Design review of the part shown in the three views and the two pictorial views. Dimensions are in mm from the part's minimum x, y and z. Coordinates: 2 decimals unless noted, no trailing zeros. Loops run counter-clockwise (first coordinate to the right, second up) from the corner with the lowest first, then second, coordinate; pieces in that order, holes last. Notation, with made-up numbers: M 65.25,41.5 L 97.25,41.5 A15 cw 97.25,55.5 Z; hole C 36.5,8.25 d8. An arc over 180 degrees is marked long. Answer as a JSON object with one key per item and string values. Group by question number.
Item 1: Insertion check: pin 1 (3 mm diameter, centred on x = 80.5, y = 5, fed in from -Z); pin 2 (3 mm diameter, centred on x = 50, y = 5, fed in from +Z). Each pin has a flat end and moves straight along its axis. Give the tip position at first contact, or say it passes through.
Item 2: Add section A-A (z = 71.5). State the section outline as (x, y) points, then the cut area to 3 significant figures.
Item 3: Add section B-B (x = 80.5). State the section outline as (y, z) points.
Item 4: Wall thickness on L1, parallel to X at y = 4.75, z = 70; L2, parallel to Y at x = 19.5, z = 8; L3, parallel to Z at x = 20, y = 5: over which ranges is each line inside the solid? List them lowest first. Write a range as from..to.
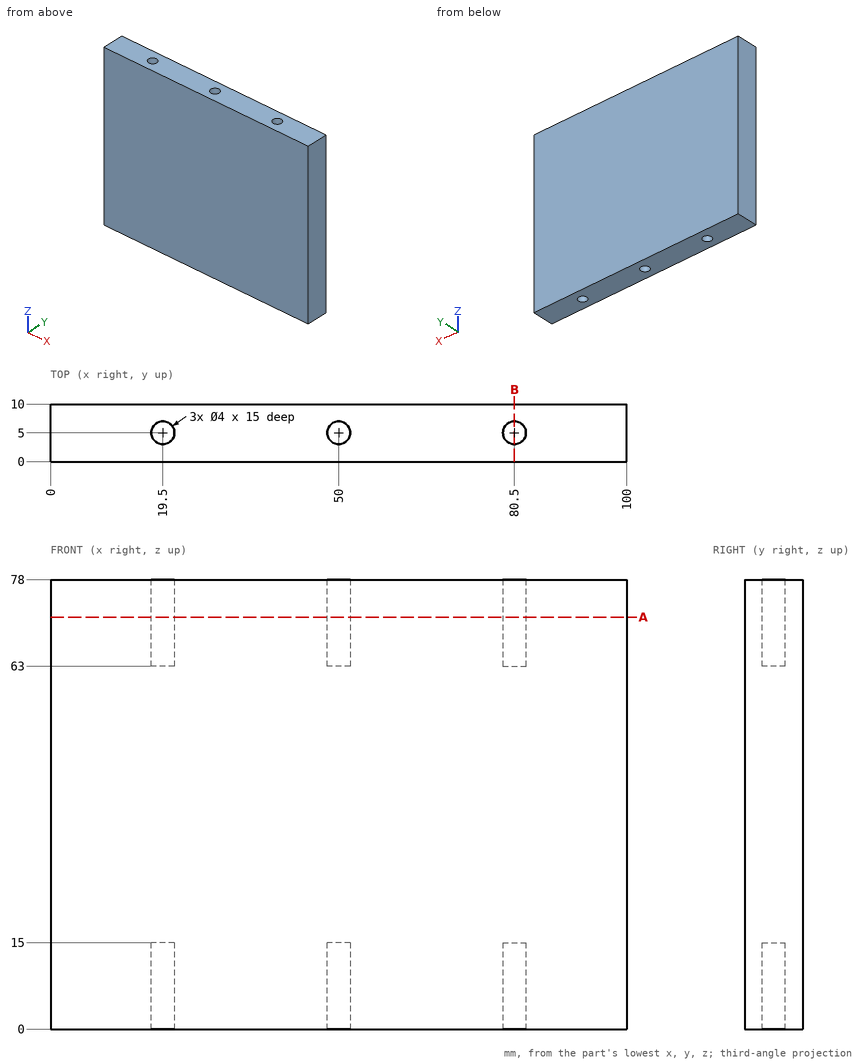
From the geometry:
{
 "1": {"pin 1": "stops at z = 15", "pin 2": "stops at z = 63"},
 "2": {"outline": "M 0,0 L 100,0 L 100,10 L 0,10 Z; hole C 19.5,5 d4; hole C 50,5 d4; hole C 80.5,5 d4", "area": "962 mm²"},
 "3": {"outline": "M 0,0 L 3,0 L 3,15 L 7,15 L 7,0 L 10,0 L 10,78 L 7,78 L 7,63 L 3,63 L 3,78 L 0,78 Z"},
 "4": {"L1": "x = 0..17.52, 21.48..48.02, 51.98..78.52, 82.48..100", "L2": "y = 0..3, 7..10", "L3": "z = 15..63"}
}
